Design review of the part built by this model. Coordinates are the model's own, in mm. A direction names the side the tool comes from. Coordinates: 2 decimals unless noted, no trailing zeros. Write each loop counter-clockwise with the first axis right and the second up, starting at its lowest first coordinate (ties: lowest second). Pieces come first, ordered by that corner, then holes. Notation, with made-up numbers: (48, 3.25) -> (85, 3.25) arc R17 cw to (85, 13.25) -> close; hole circle Ø9 at (-13, 28). An arc over 180 degrees is marked (long way). Answer in a Markdown table with one row per item. Add a question column.
Item 1: For faces 1 (the face through (-80, -4, 7.62)), 2 (the face through (-23.812, -22, 2)), 3 (the face through (-126.524, -23, 16)), list the 3-axis set-ups (+Z, -Z, +X, -X, +Y, -Y) from which the entire face can be reached by the end or side of a thin tool; tool diameter is ignored.
Item 2: Clearance check with flat-ended pins moving along their axes: P1, Ø5, axis at y = -17, z = 9, coming from the +X side; P2, Ø10, axis at y = -27, z = 22, coming from the +X side; P3, Ø3, axis at y = -32, z = 9, coming from the +X side. State where each tip first meets the part, or that it passes through.
Item 3: To check wall thickness, follow line 1 (Y direction, x = -107.5, z = 26); line 2 (Z direction, x = -65, y = -42.5); line 3 (X direction, y = -39.5, z = 20.5). State the ranges of each line that lie inside material, in increasing order.
Item 4: Draft analysis for pull direction Y (two halves, no side actions). For faces 4 (the face through (-14, -22, 0)), 5 (the face through (-80, -7.62, 28)), 6 (the face through (-97, -44.45, 26)), state which applies: released by +Y, released by -Y, zero draft, split by the parting line, or undercut.
Item 5: Take a section at A-A, the plane x = -56. Write out the cut boundary in (y, z), and give its area (3 significant figures).
from build123d import *

# Parameters (mm, degrees)
F0_W      = 177.8
F0_H      = 44.45
F1_DEPTH  = 31.75
F2_W      = 1.5875
F2_H      = 44.45
F3_DEPTH  = 3.175
F4_W      = 95.09125
F4_H      = 29.21
F5_DEPTH  = 31.751
F6_W      = 95.09125
F6_H      = 16.51
F7_DEPTH  = 44.451
F9_DEPTH  = 31.751
F11_DEPTH = 44.451


with BuildPart() as f1:
    # F0 (on Top) → F1 (new body)
    with BuildSketch(Plane.XY):
        with Locations((-88.9, -22.225)):
            Rectangle(F0_W, F0_H)
    extrude(amount=F1_DEPTH)

    # F2 (on face) → F3 (cut)
    with BuildSketch(Plane(origin=(0, 0, 0), x_dir=(1, 0, 0), z_dir=(0, 0, -1))):
        with Locations((-23.01875, 22.225)):
            Rectangle(F2_W, F2_H)
        with Locations((-134.9375, 22.225)):
            Rectangle(F2_W, F2_H)
    extrude(amount=-F3_DEPTH, mode=Mode.SUBTRACT)

    # F4 (on face) → F5 (cut, through all)
    with BuildSketch(Plane.XY.offset(31.75)):
        with Locations((-78.978125, -22.225)):
            Rectangle(F4_W, F4_H)
    extrude(amount=-F5_DEPTH, mode=Mode.SUBTRACT)

    # F6 (on face) → F7 (cut, through all)
    with BuildSketch(Plane.XZ.offset(44.45)):
        with Locations((-78.978125, 15.875)):
            Rectangle(F6_W, F6_H)
    extrude(amount=-F7_DEPTH, mode=Mode.SUBTRACT)

    # F8 (on face) → F9 (cut, through all)
    with BuildSketch(Plane.XY.offset(31.75)):
        with BuildLine():
            ThreePointArc((-14.605, 0), (-3.978035, -8.927851), (0, -22.225))
            Line((0, -22.225), (0, 0))
            Line((0, 0), (-14.605, 0))
        make_face()
        with BuildLine():
            ThreePointArc((0, -22.225), (-3.978035, -35.522149), (-14.605, -44.45))
            Line((-14.605, -44.45), (0, -44.45))
            Line((0, -44.45), (0, -22.225))
        make_face()
    extrude(amount=-F9_DEPTH, mode=Mode.SUBTRACT)

    # F10 (on face) → F11 (cut, through all)
    with BuildSketch(Plane(origin=(0, 0, 0), x_dir=(-1, 0, 0), z_dir=(0, 1, 0))):
        Polygon((0, 16.51), (23.8125, 31.75), (0, 31.75), align=None)
    extrude(amount=-F11_DEPTH, mode=Mode.SUBTRACT)


solid = f1.part
Answers:
| question | item | result |
|---|---|---|
| 1 | face 1 | +Y, -Y |
| 1 | face 2 | -Z, +Y, -Y |
| 1 | face 3 | none |
| 2 | P1 | stops at x = -0.15 |
| 2 | P2 | stops at x = -0.77 |
| 2 | P3 | stops at x = -1.46 |
| 3 | line 1 | y = -44.45 to -36.83, -7.62 to 0 |
| 3 | line 2 | z = 0 to 7.62, 24.13 to 31.75 |
| 3 | line 3 | x = -177.8 to -126.52, -31.43 to -7.25 |
| 4 | face 4 | zero draft |
| 4 | face 5 | undercut |
| 4 | face 6 | released by -Y |
| 5 | outline | (-44.45, 0) -> (-36.83, 0) -> (-36.83, 7.62) -> (-44.45, 7.62) -> close; (-44.45, 24.13) -> (-36.83, 24.13) -> (-36.83, 31.75) -> (-44.45, 31.75) -> close; (-7.62, 0) -> (0, 0) -> (0, 7.62) -> (-7.62, 7.62) -> close; (-7.62, 24.13) -> (0, 24.13) -> (0, 31.75) -> (-7.62, 31.75) -> close |
| 5 | area | 232 mm^2 |
